Source: CAD feature listing. Evaluate the final solid. Frame: model axes, mm. Give positions to 0.01 mm unless a question says otherwise; leave off trailing zeros. Loops run counter-clockwise (first coordinate to the right, second up) from the corner with the lowest first, then second, coordinate; pieces in that order, holes last. Notation, with made-up numbers: (-0.75, -28.5) - (25.25, -28.5) arc R26 ccw to (25.25, -6.5) - close; hole circle Ø9 at (58, 38.5). An arc over 180 degrees is marked (long way). Put each result on its own line as item: value.
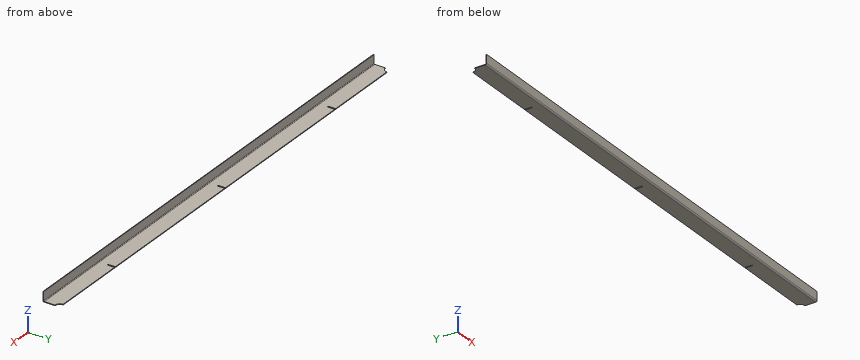
Autodesk Inventor part; units mm, degrees
ref_plane "YZ Plane" through (0, 0, 0) normal (1, 0, 0) x (0, 1, 0)
ref_plane "XZ Plane" through (0, 0, 0) normal (0, 1, 0) x (-1, 0, 0)
ref_plane "XY Plane" through (0, 0, 0) normal (0, 0, 1) x (1, 0, 0)
sketch "Sketch1" plane through (0, 0, 0) normal (0, 0, 1) x (1, 0, 0)
  line L0 (-750, 51.7458) -> (750, 51.7458)
  line L1 (750, 51.7458) -> (750, 0)
  line L2 (750, 0) -> (-750, 0)
  line L3 (-750, 0) -> (-750, 51.7458)
  point P0 (0, 0)
  point P1 (0, 0)
  dimension "d0" = 1500
  dimension "d1" = 51.7458
extrude "Plate1" add sketch "Sketch1" along normal blind 2
sketch "Sketch2" plane through (750, 2, 0) normal (0, -1, 0) x (1, 0, 0)
  line L0 (-1500, 0) -> (0, 0)
  line L1 (0, 0) -> (0, 30)
  line L2 (0, 30) -> (-1500, 30)
  line L3 (-1500, 30) -> (-1500, 0)
edge flange "Flange1" height 30 angle 90 thickness 2 bend radius 2 thickness toward (0, -1, 0) relief tear relief width 2 relief depth 1 edges at (0, 0, 2) wall of the first edge with corners at (-750, 2, 0) (750, 2, 0) (750, 2, 30) (-750, 2, 30)
bend "Bend1"
corner "Corner1"
sketch "Sketch5" plane through (0, 0, 0) normal (0, 0, -1) x (-1, 0, 0)
  line L0 (750, 51.7458) -> (-750, 51.7458)
  line L1 (498, 51.7458) -> (498, 29)
  line L2 (498, 29) -> (500, 29)
  line L3 (500, 29) -> (500, 51.7458) construction
  line L4 (750, 0) -> (-750, 0)
  line L5 (500, 29) -> (502, 29)
  line L6 (502, 29) -> (502, 51.7458)
  point P0 (0, 0)
  dimension "d18" = 2
  dimension "d19" = 250
  dimension "d20" = 29
  dimension "d27" = 2
extrude "Extrusion1" cut sketch "Sketch5" against normal through all
pattern_linear "Rectangular Pattern1" count 3 spacing 500 along (1, 0, 0) of "Extrusion1"
sketch "Sketch6" plane through (0, 0, 0) normal (0, 0, -1) x (-1, 0, 0)
  line L0 (-750, 51.7458) -> (-750, 4)
  circle A0 centre (-750, 51.7458) radius 15
  line L1 (-750, 51.7458) -> (750, 51.7458)
  point P0 (0, 0)
  point P1 (-502, 51.7458)
  point P2 (-735, 51.7458)
  point P3 (-750, 36.7458)
  dimension "d24" = 30
extrude "Extrusion2" cut sketch "Sketch6" against normal through all contours L1 A0 L0 picked at (-740.1254, 50.6332)
mirror "Mirror1" about plane through (0, 0, 0) normal (1, 0, 0) of "Extrusion2"
equation "\"d1\" = Стрингер_1"
equation "\"d18\" = Thickness"
equation "\"d27\" = d18"
equation "\"d2\" = Thickness"
equation "\"d3\" = BendReliefWidth"
equation "\"d4\" = BendReliefDepth"
equation "\"d5\" = MinimumRemnant"
equation "\"d6\" = TransitionRadius"
equation "\"d9\" = BendRadius"
equation "\"d10\" = CornerReliefSize"
equation "\"d11\" = GapSize"
equation "\"d12\" = JacobiRadiusSize"
equation "\"BendRadius\" = Thickness"
equation "\"BendReliefWidth\" = Thickness"
equation "\"BendReliefDepth\" = 0.5 * Thickness"
equation "\"CornerReliefSize\" = 4 * Thickness"
equation "\"MinimumRemnant\" = 2 * Thickness"
equation "\"TransitionRadius\" = BendRadius"
equation "\"JacobiRadiusSize\" = BendRadius"
equation "\"GapSize\" = Thickness"
equation "\"qqqqqq\" = 67.35706"
properties part number "МОО 051 стрингер спина 12" material "Stainless Steel"
1) Pin query (flat end, axial travel): P1, Ø1.6, axis at x = -500.5, z = 1, coming from the +Y side; P2, Ø1.5, axis at x = -532.5, z = 24, coming from the +Y side; P3, Ø1, axis at y = 45.5, z = 1, coming from the -X side. Return the tip coordinate at first contact, or that it passes through.
Check result:
P1: y = 29
P2: y = 2
P3: x = -736.6
2) Section query A-A, the plane x = -35.5. Output: boundary loops of the cut face in (y, z).
Check result:
outline: (0, 4) arc R4 ccw to (4, 0) - (51.75, 0) - (51.75, 2) - (4, 2) arc R2 cw to (2, 4) - (2, 30) - (0, 30) - close
3) Material intervals for line 1 along Y through (x, z) = (-362, 21.5); line 2 along Y through (x, z) = (-236.5, 2.75), sorted ascending. Write a range as [from, to].
Check result:
line 1: [0, 2]
line 2: [0.2, 2.44]
4) Section query B-B, the plane y = 14. Output: boundary loops of the cut face in (x, z).
Check result:
outline: (-750, 0) - (750, 0) - (750, 2) - (-750, 2) - close
